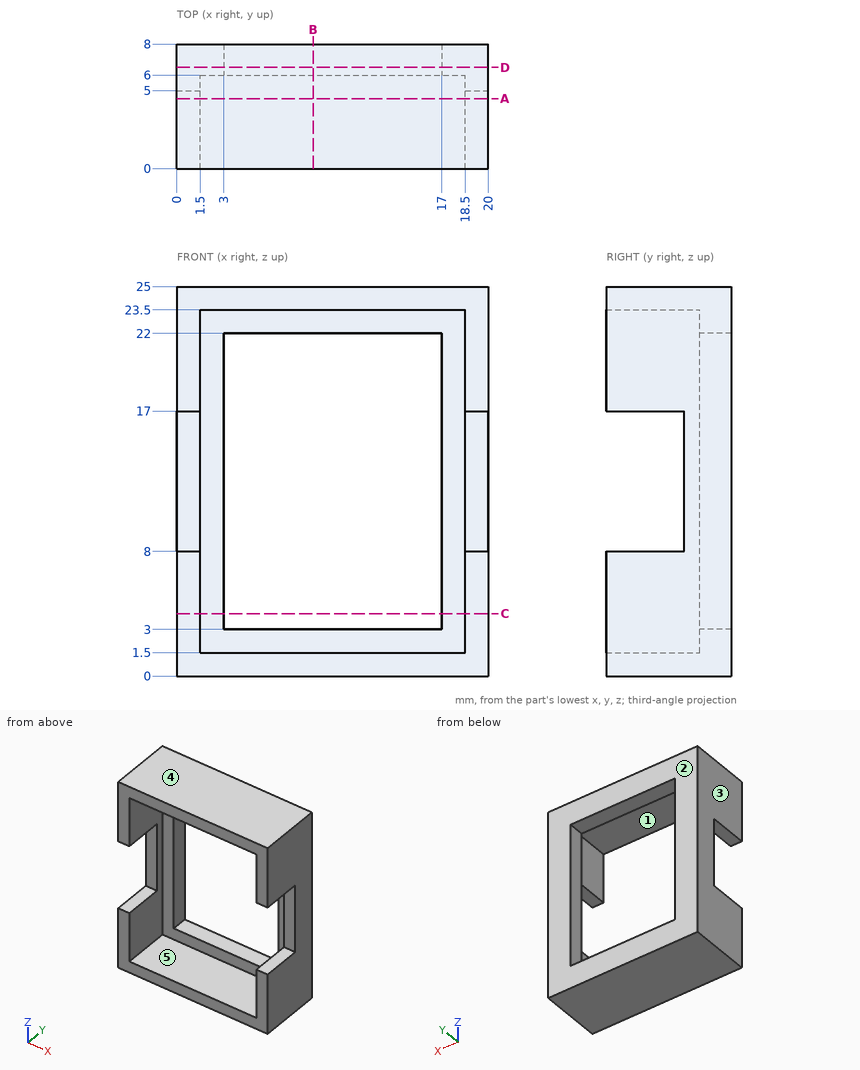
Part print with two shaded views. Sizes in mm from the minimum x, y, z corner. A direction names the side the tool comes from. Give positions to 0.01 mm unless a question says otherwise; leave off trailing zeros. Write each loop counter-clockwise with the first axis right and the second up, starting at its lowest first coordinate (ties: lowest second). Pieces come first, ordered by that corner, then holes.
1) Cut at B-B on x = 8.75. Write the cut outline in (y, z).
Resolved:
outline: (0, 0) - (8, 0) - (8, 3) - (6, 3) - (6, 1.5) - (0, 1.5) - close; (0, 23.5) - (6, 23.5) - (6, 22) - (8, 22) - (8, 25) - (0, 25) - close
2) Pin check, flat tips, straight feed: pin 1 (1.6 mm diameter, centred on x = 1, z = 10.5, fed in from -Y); pin 2 (1 mm diameter, centred on y = 3, z = 9.5, fed in from +X). Stop position of each tip, or through.
Resolved:
pin 1: stops at y = 5
pin 2: passes through
3) Which spindle directions (+Z, -Z, +X, -X, +Y, -Y) get a long thin tool onto all of the face, cutting with end or side? Do the marked faces 1 and 2. Say none if no direction does.
Resolved:
face 1: -Y
face 2: +Z, -Z, +X, -X, +Y
4) Cut at D-D on y = 6.5. Write the cut outline in (x, z), then the cut area to 3 significant figures.
Resolved:
outline: (0, 0) - (20, 0) - (20, 25) - (0, 25) - close; hole (3, 3) - (17, 3) - (17, 22) - (3, 22) - close
area: 234 mm2
5) Two-plate mould, pull along Z, no slides. Class the marked faces 3, 4 and 5: released by +Z, released by -Z, zero draft, split by the parting line, or undercut.
Resolved:
face 3: zero draft
face 4: released by +Z
face 5: undercut
6) Cut at A-A on y = 4.5. Write the cut outline in (x, z).
Resolved:
outline: (0, 0) - (20, 0) - (20, 8) - (18.5, 8) - (18.5, 1.5) - (1.5, 1.5) - (1.5, 8) - (0, 8) - close; (0, 17) - (1.5, 17) - (1.5, 23.5) - (18.5, 23.5) - (18.5, 17) - (20, 17) - (20, 25) - (0, 25) - close
7) Cut at C-C on z = 4. Write the cut outline in (x, y), then the cut area to 3 significant figures.
Resolved:
outline: (0, 0) - (1.5, 0) - (1.5, 6) - (3, 6) - (3, 8) - (0, 8) - close; (17, 6) - (18.5, 6) - (18.5, 0) - (20, 0) - (20, 8) - (17, 8) - close
area: 30.0 mm2
8) Probe L1, parallel to Z at x = 16.5, y = 2.75; L2, parallel to X at y = 7.25, z = 14; L3, parallel to X at y = 1.5, z = 19.75. List the from-to ranges inside material, lowest first.
Resolved:
L1: z = 0 to 1.5, 23.5 to 25
L2: x = 0 to 3, 17 to 20
L3: x = 0 to 1.5, 18.5 to 20
